Input: part model. Units: mm. Frame: model coordinates. Coordinates: 2 decimals unless noted, no trailing zeros. Loops run counter-clockwise (first coordinate to the right, second up) from the corner with the lowest first, then second, coordinate; pieces in that order, holes last. Notation, with made-up numbers: (-11.75, 11.5) - (46.25, 11.5) arc R9 ccw to (46.25, 15.5) - close; hole circle Ø6 at (2.5, 46.5). An arc over 180 degrees is marked (long way). Use one line per item in the form item = value.
Autodesk Inventor part; units mm, degrees
ref_plane "YZ Plane" through (0, 0, 0) normal (1, 0, 0) x (0, 1, 0)
ref_plane "XZ Plane" through (0, 0, 0) normal (0, 1, 0) x (-1, 0, 0)
ref_plane "XY Plane" through (0, 0, 0) normal (0, 0, 1) x (1, 0, 0)
sketch "Sketch1" plane through (0, 0, 0) normal (0, 0, 1) x (1, 0, 0)
  circle A0 centre (0, 0) radius 4.445
  dimension "d1" = 8.89
extrude "Extrusion1" add sketch "Sketch1" along normal mid plane 90.6272
sketch "Sketch2" plane through (0, 0, 45.3136) normal (0, 0, 1) x (1, 0, 0)
  point P0 (0, 0)
hole "Hole1" at (0, 0, 45.3136) direction (0, 0, -1) diameter 3.683 depth 37.9984 tip angle 118
thicken "Thicken1" operation add thickness 23.0632 both sides no extend neighbours yes toward (0, 0, -1) faces at (3.5296, -0.4286, 45.3136)
properties part number "drive train standoff"
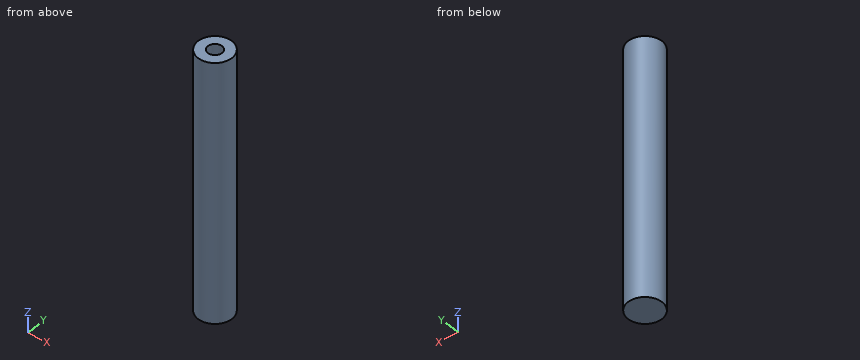
Q1. Cut plane B-B, the plane z = -18. Return loops of the section in (x, y) (3 decimals).
Check values:
outline = circle Ø8.89 at (0, 0)
Q2. Cut plane C-C, the plane x = 3.25. Return loops of the section in (y, z).
Check values:
outline = (-3.03, -45.31) - (3.03, -45.31) - (3.03, 22.25) - (-3.03, 22.25) - close
Q3. First-contact query: P1, Ø5, axis at x = -3.5, z = 11.5, coming from the -Y side; P2, Ø2, axis at x = -2, z = -9, coming from the +Y side; P3, Ø2, axis at x = 3.5, z = 6, coming from the -Y side. Flat tips, straight axial feed; report the tip coordinate or a pass-through.
Check values:
P1 = -4.33
P2 = 4.33
P3 = -3.68
Q4. Cut plane A-A, the plane z = 8. Return loops of the section in (x, y) (1 decimal), then the cut area to 3 significant figures.
Check values:
outline = circle Ø8.9 at (0, 0); hole circle Ø3.7 at (0, 0)
area = 51.4 mm²
